```python
from build123d import *

# Parameters (mm, degrees)
F0_R     = 6.35
F1_DEPTH = 12.7


with BuildPart() as f1:
    # F0 (on Top) → F1 (new body)
    with BuildSketch(Plane.XY):
        Polygon((-11.073005, 20.208511), (-36.473005, 20.208511), (-36.473005, -30.591489), (65.126995, -30.591489), (65.126995, -5.191489), (14.326995, -5.191489), (14.326995, 7.508511), (1.626995, 7.508511), (1.626995, -5.191489), (-11.073005, -5.191489), align=None)
        with Locations((-23.773005, 7.508511)):
            Circle(F0_R, mode=Mode.SUBTRACT)
    extrude(amount=F1_DEPTH)


solid = f1.part
```
CAD build for the part. Positions are in the model's coordinates, mm. A direction names the side the tool comes from. Coordinates: 2 decimals unless noted, no trailing zeros. Order: outer loops, then holes, each group sorted by start corner. A loop starts at its lowest first (then second) coordinate and runs counter-clockwise, first axis right, second up. Notation, with made-up numbers: (89.5, 74.25) -> (102.5, 74.25) arc R18 ccw to (102.5, 82.25) -> close; hole circle Ø7 at (85, -33.75). An arc over 180 degrees is marked (long way). Use one line per item in the form item = value. Start each with the question number.
1) Pull direction Y, two halves, no side cores. Call faces 4 (the flat face through (-11.073, 7, 6)), 5 (the flat face through (-5, -5.191, 6)), 6 (the cylindrical face through (-25.1, 1.3, 6.3)), 7 (the flat face through (14, -30.591, 6)): +Y half, -Y half, draft (parallel to the pull), parting line (faces both ways), or undercut.
2) Band-saw the part on B-B on z = 2. Give the cut face in (x, y), then the cut area to 3 significant figures.
3) Drill centre lines: L1, parallel to Y at x = 0, z = 11.25; L2, parallel to X at y = 8, z = 2.75; L3, parallel to X at y = 3, z = 10.25. Where is each one in solid material? Low to high. Write a range as [from, to].
4) Tool access for faces 1 (the flat face through (2, -10, 12.7)), 2 (the flat face through (8, 7.509, 6)), 3 (the flat face through (1.627, 1, 6)): list every direction of +Z, -Z, +X, -X, +Y, -Y with a clear straight run to the whole face (end or side of a thin tool).
5) Drop flat-ended pins along their axis: pin 1 (6.5 mm diameter, centred on x = 6, z = 6, fed in from +Y); pin 2 (6 mm diameter, centred on x = 43, z = 7.5, fed in from +Y); pin 3 (4 mm diameter, centred on y = 4, z = 5.5, fed in from +X). Give the stop position or say it passes through.
6) Band-saw the part on C-C on y = 5. Give the cut face in (x, z), then the cut area to 3 significant figures.
7) Band-saw the part on A-A on y = -2. Give the cut face in (x, z).
8) Band-saw the part on D-D on x = 9. Give the cut face in (y, z), then the cut area to 3 significant figures.
Entries:
q1.face_4 = draft
q1.face_5 = +Y half
q1.face_6 = undercut
q1.face_7 = -Y half
q2.outline = (-36.47, -30.59) -> (65.13, -30.59) -> (65.13, -5.19) -> (14.33, -5.19) -> (14.33, 7.51) -> (1.63, 7.51) -> (1.63, -5.19) -> (-11.07, -5.19) -> (-11.07, 20.21) -> (-36.47, 20.21) -> close; hole circle Ø12.7 at (-23.77, 7.51)
q2.area = 3,260 mm2
q3.L1 = [-30.59, -5.19]
q3.L2 = [-36.47, -30.1], [-17.44, -11.07]
q3.L3 = [-36.47, -28.24], [-19.3, -11.07], [1.63, 14.33]
q4.face_1 = +Z, +X, -X, +Y, -Y
q4.face_2 = +Z, -Z, +X, +Y
q4.face_3 = +Z, -Z, +Y
q5.pin_1 = 7.51
q5.pin_2 = -5.19
q5.pin_3 = 14.33
q6.outline = (-36.47, 0) -> (-29.61, 0) -> (-29.61, 12.7) -> (-36.47, 12.7) -> close; (-17.94, 0) -> (-11.07, 0) -> (-11.07, 12.7) -> (-17.94, 12.7) -> close; (1.63, 0) -> (14.33, 0) -> (14.33, 12.7) -> (1.63, 12.7) -> close
q6.area = 336 mm2
q7.outline = (-36.47, 0) -> (-11.07, 0) -> (-11.07, 12.7) -> (-36.47, 12.7) -> close; (1.63, 0) -> (14.33, 0) -> (14.33, 12.7) -> (1.63, 12.7) -> close
q8.outline = (-30.59, 0) -> (7.51, 0) -> (7.51, 12.7) -> (-30.59, 12.7) -> close
q8.area = 484 mm2
